from build123d import *

# Parameters (mm, degrees)
F0_W     = 6.2131884992
F0_H     = 3.9810055999
F1_DEPTH = 13


with BuildPart() as f1:
    # F0 (on Top) → F1 (new body)
    with BuildSketch(Plane.XY):
        Polygon((-60.5168718398, 57.2218040137), (-64.5168718398, 57.2218040137), (-64.5168718398, 40.2218040137), (-60.5168718398, 40.2218040137), (-60.5168718398, 53.2407984138), align=None)
        with Locations((-57.4102775902, 55.2313012137)):
            Rectangle(F0_W, F0_H)
    extrude(amount=F1_DEPTH)


solid = f1.part
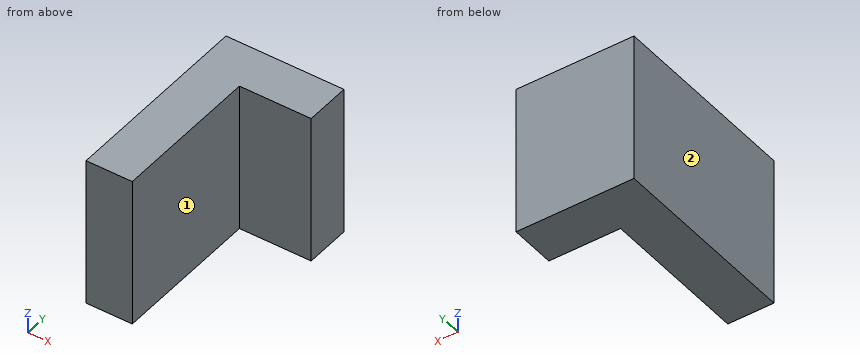
Check sheet for the modelled part. Datum: model origin and axes. Units: mm. Face numbers are marked on the shaded views. A direction names the side the tool comes from. Give positions to 0.01 mm unless a question says otherwise; leave off trailing zeros. Write each loop counter-clockwise with the first axis right and the second up, starting at its lowest first coordinate (ties: lowest second). Pieces come first, ordered by that corner, then holes. Notation, with made-up numbers: M 81.25,34.5 L 90.25,34.5 A23 cw 90.25,56.5 Z; hole C 11.25,17.5 d3. An arc over 180 degrees is marked long. Use one line per item in the form item = value.
(1) Material ranges on line 1 along Y through (x, z) = (-55, 8.5); line 2 along X through (y, z) = (43.75, 8.5), recorded low to high.
Answer block:
line_1 = 53.24 to 57.22
line_2 = -64.52 to -60.52
(2) Section check A-A on z = 1. Record the boundary of the cut face in (x, y), plus the area to 3 significant figures.
Answer block:
outline = M -64.52,40.22 L -60.52,40.22 L -60.52,53.24 L -54.3,53.24 L -54.3,57.22 L -64.52,57.22 Z
area = 92.7 mm2
(3) Section check B-B on x = -56.25. Record the boundary of the cut face in (y, z), plus the area to 3 significant figures.
Answer block:
outline = M 53.24,0 L 57.22,0 L 57.22,13 L 53.24,13 Z
area = 51.8 mm2
(4) Section check C-C on y = 51. Record the boundary of the cut face in (x, z), plus the area to 3 significant figures.
Answer block:
outline = M -64.52,0 L -60.52,0 L -60.52,13 L -64.52,13 Z
area = 52.0 mm2
(5) Tool access check on the marked faces 1 and 2. Record the directions out of +Z, -Z, +X, -X, +Y, -Y that give a thin tool (end or side, any length) a straight path to the whole face; none if there is none.
Answer block:
face_1 = +Z, -Z, +X, -Y
face_2 = +Z, -Z, -X, +Y, -Y
(6) Depth check by flat-ended pin: P1, Ø1, axis at y = 47, z = 9, coming from the +X side. Enter the tip coordinate at first touch or a pass-through.
Answer block:
P1 = -60.52
